Design review of the part built by this model. Coordinates are the model's own, in mm. Give positions to 0.01 mm unless a question says otherwise; leave off trailing zeros. Loops run counter-clockwise (first coordinate to the right, second up) from the corner with the lowest first, then second, coordinate; pieces in that order, holes last.
from build123d import *

# Parameters (mm, degrees)
SKETCH_1_R      = 1.75
EXTRUDE_1_DEPTH = 5


with BuildPart() as part:
    # Эскиз1 → Бобышка-Вытянуть1 (new body)
    with BuildSketch(Plane.XY):
        with BuildLine():
            Line((-48, -50), (48, -50))
            ThreePointArc((48, -50), (49.414213562, -49.414213562), (50, -48))
            Line((50, -48), (50, 48))
            ThreePointArc((50, 48), (49.414213562, 49.414213562), (48, 50))
            Line((48, 50), (-48, 50))
            ThreePointArc((-48, 50), (-49.414213562, 49.414213562), (-50, 48))
            Line((-50, 48), (-50, -48))
            ThreePointArc((-50, -48), (-49.414213562, -49.414213562), (-48, -50))
        make_face()
        with Locations((-47, 35)):
            Circle(SKETCH_1_R, mode=Mode.SUBTRACT)
        with Locations((47, 35)):
            Circle(SKETCH_1_R, mode=Mode.SUBTRACT)
        with Locations((47, -35)):
            Circle(SKETCH_1_R, mode=Mode.SUBTRACT)
        with Locations((-47, -35)):
            Circle(SKETCH_1_R, mode=Mode.SUBTRACT)
        with Locations((-35, 47)):
            Circle(SKETCH_1_R, mode=Mode.SUBTRACT)
        with Locations((35, 47)):
            Circle(SKETCH_1_R, mode=Mode.SUBTRACT)
        with Locations((-35, -47)):
            Circle(SKETCH_1_R, mode=Mode.SUBTRACT)
        with Locations((35, -47)):
            Circle(SKETCH_1_R, mode=Mode.SUBTRACT)
        with Locations((-10, 40)):
            Circle(SKETCH_1_R, mode=Mode.SUBTRACT)
        with Locations((12, 40)):
            Circle(SKETCH_1_R, mode=Mode.SUBTRACT)
        with Locations((-10, -35)):
            Circle(SKETCH_1_R, mode=Mode.SUBTRACT)
        with Locations((12, -35)):
            Circle(SKETCH_1_R, mode=Mode.SUBTRACT)
    extrude(amount=EXTRUDE_1_DEPTH)


solid = part.part
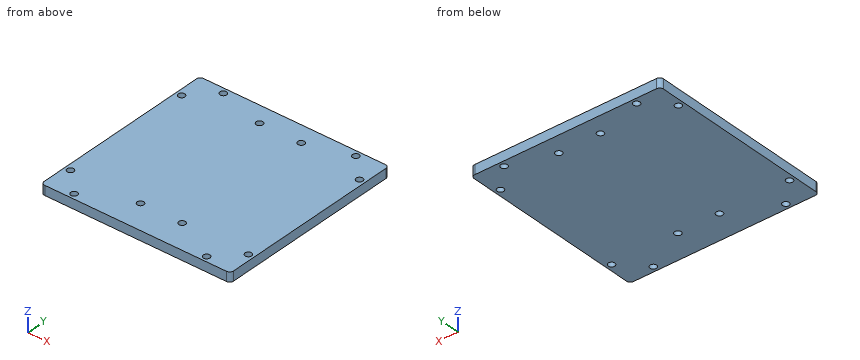
Q1. Take a section at C-C (y = 40). Give the boundary of the cut face in (x, z).
Results:
outline: (-50, 0) - (-11.75, 0) - (-11.75, 5) - (-50, 5) - close; (-8.25, 0) - (10.25, 0) - (10.25, 5) - (-8.25, 5) - close; (13.75, 0) - (50, 0) - (50, 5) - (13.75, 5) - close
Q2. Insertion check: pin 1 (4 mm diameter, centred on x = 47, y = -35, fed in from +Z); pin 2 (3 mm diameter, centred on x = 35, y = -47, fed in from -Z). Each pin has a flat end and moves straight along its axis. Give the tip position at first contact, or say it passes through.
Results:
pin 1: stops at z = 5
pin 2: passes through
Q3. Wall thickness on line 1 (Y direction, x = 35, z = 2.75); line 2 (Y direction, x = -47, z = 2.2); line 3 (X direction, y = -35.5, z = 2.5): over which ranges is each line inside the solid? List them lowest first.
Results:
line 1: y = -50 to -48.75, -45.25 to 45.25, 48.75 to 50
line 2: y = -50 to -36.75, -33.25 to 33.25, 36.75 to 50
line 3: x = -50 to -48.68, -45.32 to -11.68, -8.32 to 10.32, 13.68 to 45.32, 48.68 to 50
Q4. Take a section at A-A (x = 35). Give the boundary of the cut face in (y, z), plus the area to 3 significant figures.
Results:
outline: (-50, 0) - (-48.75, 0) - (-48.75, 5) - (-50, 5) - close; (-45.25, 0) - (45.25, 0) - (45.25, 5) - (-45.25, 5) - close; (48.75, 0) - (50, 0) - (50, 5) - (48.75, 5) - close
area: 465 mm2
Q5. Take a section at B-B (y = -35). Give the boundary of the cut face in (x, z), plus the area to 3 significant figures.
Results:
outline: (-50, 0) - (-48.75, 0) - (-48.75, 5) - (-50, 5) - close; (-45.25, 0) - (-11.75, 0) - (-11.75, 5) - (-45.25, 5) - close; (-8.25, 0) - (10.25, 0) - (10.25, 5) - (-8.25, 5) - close; (13.75, 0) - (45.25, 0) - (45.25, 5) - (13.75, 5) - close; (48.75, 0) - (50, 0) - (50, 5) - (48.75, 5) - close
area: 430 mm2
